Verification items for the finished model (mm, model axes). A direction names the side the tool comes from. Coordinates: 2 decimals unless noted, no trailing zeros. Order: outer loops, then holes, each group sorted by start corner. A loop starts at its lowest first (then second) coordinate and runs counter-clockwise, first axis right, second up. Notation, with made-up numbers: M 27.5,54 L 46.5,54 A18 ccw 46.5,68 Z; hole C 89.25,-21 d11. An arc over 180 degrees is marked long. Return JSON: item names as keys, results as strings.
```python
from build123d import *

# Parameters (mm, degrees)
F2_DEPTH = 20
F3_R     = 12.5
F4_DEPTH = 25


with BuildPart() as f2:
    # F1 (on Top) → F2 (new body)
    with BuildSketch(Plane.XY):
        with BuildLine():
            ThreePointArc((22.9128784748, -10), (24.4726578233, -5.1077410922), (25, 0))
            ThreePointArc((25, 0), (24.4726578233, 5.1077410922), (22.9128784748, 10))
            Line((22.9128784748, 10), (22.9128784748, 0))
            Line((22.9128784748, 0), (22.9128784748, -10))
        make_face()
        with BuildLine():
            ThreePointArc((22.9128784748, 10), (24.4726578233, 5.1077410922), (25, 0))
            ThreePointArc((25, 0), (24.4726578233, -5.1077410922), (22.9128784748, -10))
            Line((22.9128784748, -10), (52.9128784748, -10))
            Line((52.9128784748, -10), (52.9128784748, 10))
            Line((52.9128784748, 10), (22.9128784748, 10))
        make_face()
        with BuildLine():
            Line((22.9128784748, 0), (22.9128784748, 10))
            ThreePointArc((22.9128784748, 10), (9.5670858091, 23.0969883128), (-9.1307839342, 23.2729195579))
            Line((-9.1307839342, 23.2729195579), (-23.2729195579, 9.1307839342))
            ThreePointArc((-23.2729195579, 9.1307839342), (-25, 0), (-23.2729195579, -9.1307839342))
            Line((-23.2729195579, -9.1307839342), (-9.1307839342, -23.2729195579))
            ThreePointArc((-9.1307839342, -23.2729195579), (9.5670858091, -23.0969883128), (22.9128784748, -10))
            Line((22.9128784748, -10), (22.9128784748, 0))
        make_face()
        with BuildLine():
            Line((-23.2729195579, 9.1307839342), (-9.1307839342, 23.2729195579))
            ThreePointArc((-9.1307839342, 23.2729195579), (-17.6776695297, 17.6776695297), (-23.2729195579, 9.1307839342))
        make_face()
        with BuildLine():
            ThreePointArc((-23.2729195579, 9.1307839342), (-17.6776695297, 17.6776695297), (-9.1307839342, 23.2729195579))
            Line((-9.1307839342, 23.2729195579), (-30.3439873698, 44.4861229935))
            Line((-30.3439873698, 44.4861229935), (-37.4150551816, 37.4150551816))
            Line((-37.4150551816, 37.4150551816), (-44.4861229935, 30.3439873698))
            Line((-44.4861229935, 30.3439873698), (-23.2729195579, 9.1307839342))
        make_face()
        with BuildLine():
            Line((-30.3439873698, -44.4861229935), (-9.1307839342, -23.2729195579))
            ThreePointArc((-9.1307839342, -23.2729195579), (-17.6776695297, -17.6776695297), (-23.2729195579, -9.1307839342))
            Line((-23.2729195579, -9.1307839342), (-44.4861229935, -30.3439873698))
            Line((-44.4861229935, -30.3439873698), (-37.4150551816, -37.4150551816))
            Line((-37.4150551816, -37.4150551816), (-30.3439873698, -44.4861229935))
        make_face()
        with BuildLine():
            ThreePointArc((-23.2729195579, -9.1307839342), (-17.6776695297, -17.6776695297), (-9.1307839342, -23.2729195579))
            Line((-9.1307839342, -23.2729195579), (-23.2729195579, -9.1307839342))
        make_face()
    extrude(amount=F2_DEPTH)

    # F3 (on face) → F4 (cut)
    with BuildSketch(Plane.XY.offset(20)):
        Circle(F3_R)
    extrude(amount=-F4_DEPTH, mode=Mode.SUBTRACT)


solid = f2.part
```
Q1. Cross-section at C-C, the plane z = 13.25. Record the boundary of the cut face in (x, y), and give its area (3 significant figures).
Values:
{"outline": "M -44.49,-30.34 L -30.34,-44.49 L -9.13,-23.27 A25 ccw 22.91,-10 L 52.91,-10 L 52.91,10 L 22.91,10 A25 ccw -9.13,23.27 L -30.34,44.49 L -44.49,30.34 L -23.27,9.13 A25 ccw -23.27,-9.13 Z; hole C 0,0 d25", "area": "3,190 mm^2"}
Q2. Cross-section at D-D, the plane x = 28.5. Record the boundary of the cut face in (y, z).
Values:
{"outline": "M -10,0 L 10,0 L 10,20 L -10,20 Z"}
Q3. Material ranges on line 1 along Y through (x, z) = (0, 12.25); line 2 along Y through (x, z) = (-38, 1); line 3 along X through (y, z) = (-5, 9.5), recorded low to high.
Values:
{"line 1": "-25 to -12.5, 12.5 to 25", "line 2": "-36.83 to -23.86, 23.86 to 36.83", "line 3": "-24.49 to -11.46, 11.46 to 52.91"}
Q4. Cross-section at B-B, the plane y = 0. Record the boundary of the cut face in (x, z), and give its area (3 significant figures).
Values:
{"outline": "M -25,0 L -12.5,0 L -12.5,20 L -25,20 Z; M 12.5,0 L 52.91,0 L 52.91,20 L 12.5,20 Z", "area": "1,060 mm^2"}
Q5. Draft check along X on faces 1 (the face through (9.319, -23.198, 9.86)), 2 (the face through (-7, 11, 20)), 3 (the face through (11.923, 3.755, 10.14)), 4 (the face through (-34.03, 19.89, 9.86)). Enter one of: pulls with the +X half, pulls with the -X half, needs draft (parallel to the pull), parting line crosses it, or undercut.
Values:
{"face 1": "undercut", "face 2": "needs draft", "face 3": "undercut", "face 4": "pulls with the -X half"}
Q6. Cross-section at A-A, the plane x = 0. Record the boundary of the cut face in (y, z).
Values:
{"outline": "M -25,0 L -12.5,0 L -12.5,20 L -25,20 Z; M 12.5,0 L 25,0 L 25,20 L 12.5,20 Z"}
Q7. Go/stop test with flat-tipped pins: pin 1 (6 mm diameter, centred on x = 42, z = 11.5, fed in from +Y); pin 2 (10 mm diameter, centred on x = 32, z = 11, fed in from -Y); pin 3 (1.5 mm diameter, centred on x = 1.5, z = 6, fed in from -Y). Record where each tip stops, or that it passes through.
Values:
{"pin 1": "y = 10", "pin 2": "y = -10", "pin 3": "y = -24.99"}
Q8. Tool access check on faces 5 (the face through (38, 10, 10)), 6 (the face through (-33.73, -19.59, 9.86)), 7 (the face through (38, -10, 10)). Record the directions out of +Z, -Z, +X, -X, +Y, -Y that give a thin tool (end or side, any length) a straight path to the whole face; none if there is none.
Values:
{"face 5": "+Z, -Z, +X, +Y", "face 6": "+Z, -Z, -X", "face 7": "+Z, -Z, +X, -Y"}
